Design review of the part built by this model. Coordinates are the model's own, in mm. A direction names the side the tool comes from. Give positions to 0.01 mm unless a question says otherwise; leave off trailing zeros. Write each loop counter-clockwise with the first axis right and the second up, starting at its lowest first coordinate (ties: lowest second). Pieces come first, ordered by that corner, then holes. Notation, with made-up numbers: M 86.25,16 L 120.25,16 A35 cw 120.25,52 Z; hole C -17,-1.75 d10. An arc over 180 degrees is marked long. Write each question's results on one line, items separated by ' | '. Start each with the question number.
from build123d import *

# Parameters (mm, degrees)
SKETCH1_W           = 10
SKETCH1_H           = 6
BOSS_EXTRUDE1_DEPTH = 1.8
BOSS_EXTRUDE2_DEPTH = 5.2
BOSS_EXTRUDE3_START = -5
SKETCH3_W           = 0.6
SKETCH3_H           = 0.6
BOSS_EXTRUDE3_DEPTH = 9.2
LPATTERN1_COUNT     = 3
LPATTERN1_PITCH     = 2.54


with BuildPart() as part:
    # Sketch1 → Boss-Extrude1 (new body)
    with BuildSketch(Plane.XY):
        Rectangle(SKETCH1_W, SKETCH1_H)
    extrude(amount=BOSS_EXTRUDE1_DEPTH)

    # Sketch2 → Boss-Extrude2 (add)
    with BuildSketch(Plane.XY.offset(1.8)):
        Polygon((-2, -3), (-2, -2.4), (-4.4, -2.4), (-4.4, 2.4), (4.4, 2.4), (4.4, -2.4), (2, -2.4), (2, -3), (5, -3), (5, 3), (-5, 3), (-5, -3), align=None)
    extrude(amount=BOSS_EXTRUDE2_DEPTH)

    # Sketch3 → Boss-Extrude3 (add)
    with BuildSketch(Plane.XY.offset(1.8).offset(BOSS_EXTRUDE3_START)):
        with Locations((-2.54, -0.5)):
            Rectangle(SKETCH3_W, SKETCH3_H)
    boss_extrude3 = extrude(amount=BOSS_EXTRUDE3_DEPTH)

    # LPattern1: Boss-Extrude3 ×3
    with Locations(*[(i * LPATTERN1_PITCH, 0, 0) for i in range(1, LPATTERN1_COUNT)]):
        add(boss_extrude3)


solid = part.part
Q1. Wall thickness on line 1 along X through (y, z) = (-0.75, 2); line 2 along X through (y, z) = (-0.75, -1); line 3 along Y through (x, z) = (4, 5): over which ranges is each line inside the solid? List them lowest first. Write a range as from..to.
Q2. For faces 1 (the flat face through (0.3, 2.7, 7)), 2 (the flat face through (4.4, 0, 4)), list the 3-axis set-ups (+Z, -Z, +X, -X, +Y, -Y) from which the entire face can be reached by the end or side of a thin tool; tool diameter is ignored.
Q3. We need section D-D on y = 1.7. Write out the cut boundary in (x, z).
Q4. We need section B-B on z = 5. Write out the cut boundary in (x, y), and give its area (3 significant figures).
Q5. We need section C-C on x = -4. Write out the cut boundary in (y, z), and give its area (3 significant figures).
Q6. We need section A-A on z = -2.5. Write out the cut boundary in (x, y).
Q7. The part is to be moulded in two halves that separate along Y. For faces 3 (the flat face through (-4.4, 0, 4)), 4 (the flat face through (0, 0, 0)), 5 (the flat face through (0, -3, 1)), say which applies: pulls with the +Y half, pulls with the -Y half, needs draft (parallel to the pull), parting line crosses it, or undercut.
Q8. For pin 1 Ø0.5 at (x, z) = (0, -1.5) entering from +Y; pin 2 Ø1 at (x, y) = (-1.5, 0.5) entering from +Z; pin 3 Ø0.7 at (x, y) = (-2.5, -0.5) entering from +Z, all flat-tipped, find the tip position at first contact; note any pin that passes through.
Answer sheet:
1) line 1: -5..-4.4, -2.84..-2.24, -0.3..0.3, 2.24..2.84, 4.4..5 | line 2: -2.84..-2.24, -0.3..0.3, 2.24..2.84 | line 3: -3..-2.4, 2.4..3
2) face 1: +Z, +X, -X, +Y, -Y | face 2: +Z
3) outline: M -5,0 L 5,0 L 5,7 L 4.4,7 L 4.4,1.8 L -4.4,1.8 L -4.4,7 L -5,7 Z
4) outline: M -5,-3 L -2,-3 L -2,-2.4 L -4.4,-2.4 L -4.4,2.4 L 4.4,2.4 L 4.4,-2.4 L 2,-2.4 L 2,-3 L 5,-3 L 5,3 L -5,3 Z; M -2.84,-0.8 L -2.24,-0.8 L -2.24,-0.2 L -2.84,-0.2 Z; M -0.3,-0.8 L 0.3,-0.8 L 0.3,-0.2 L -0.3,-0.2 Z; M 2.24,-0.8 L 2.84,-0.8 L 2.84,-0.2 L 2.24,-0.2 Z | area: 16.4 mm^2
5) outline: M -3,0 L 3,0 L 3,7 L 2.4,7 L 2.4,1.8 L -2.4,1.8 L -2.4,7 L -3,7 Z | area: 17.0 mm^2
6) outline: M -2.84,-0.8 L -2.24,-0.8 L -2.24,-0.2 L -2.84,-0.2 Z; M -0.3,-0.8 L 0.3,-0.8 L 0.3,-0.2 L -0.3,-0.2 Z; M 2.24,-0.8 L 2.84,-0.8 L 2.84,-0.2 L 2.24,-0.2 Z
7) face 3: undercut | face 4: needs draft | face 5: pulls with the -Y half
8) pin 1: y = -0.2 | pin 2: z = 1.8 | pin 3: z = 6
